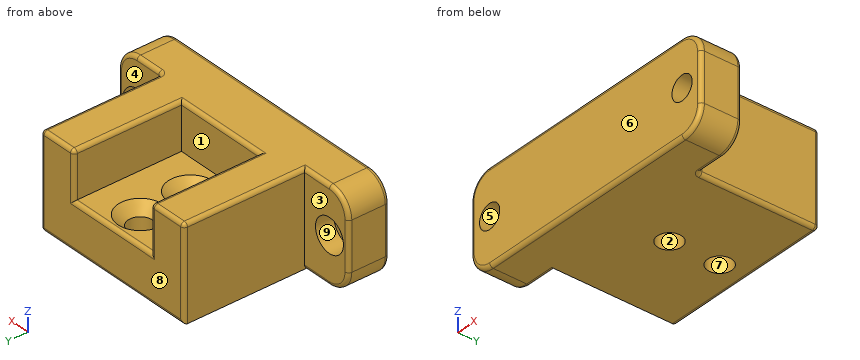
from build123d import *

# Parameters (mm, degrees)
BOSS_EXTRUDE1_DEPTH = 50
SKETCH2_W           = 50
SKETCH2_H           = 25
CUT_EXTRUDE2_DEPTH  = 58
SKETCH3_R           = 6.5
CUT_EXTRUDE3_DEPTH  = 58
SKETCH3_3_R         = 9
SKETCH3_3_R_2       = 6.5
CUT_EXTRUDE4_DEPTH  = 10
SKETCH6_R           = 6.5
CUT_EXTRUDE5_DEPTH  = 19.5
CUT_EXTRUDE9_START  = -19.5
SKETCH6_3_R         = 6.5
CUT_EXTRUDE9_DEPTH  = 8.5
CUT_EXTRUDE9_TAPER  = -45
FILLET1_R           = 12
FILLET2_R           = 2


with BuildPart() as part:
    # Sketch1 → Boss-Extrude1 (new body)
    with BuildSketch(Plane.XY):
        Polygon((74, 0), (-74, 0), (-74, 22), (-46, 22), (-46, 87), (46, 87), (46, 22), (74, 22), align=None)
    extrude(amount=BOSS_EXTRUDE1_DEPTH)

    # Sketch2 → Cut-Extrude2 (cut)
    with BuildSketch(Plane(origin=(0, 87, 0), x_dir=(1, 0, 0), z_dir=(0, 1, 0))):
        with Locations((0, -37.5)):
            Rectangle(SKETCH2_W, SKETCH2_H)
    extrude(amount=-CUT_EXTRUDE2_DEPTH, mode=Mode.SUBTRACT)

    # Sketch3 → Cut-Extrude3 (cut)
    with BuildSketch(Plane(origin=(0, 22, 0), x_dir=(1, 0, 0), z_dir=(0, 1, 0))):
        with Locations((62, -25)):
            Circle(SKETCH3_R)
    cut_extrude3 = extrude(amount=-CUT_EXTRUDE3_DEPTH, mode=Mode.SUBTRACT)

    # Sketch3_3 → Cut-Extrude4 (cut)
    with BuildSketch(Plane(origin=(0, 22, 0), x_dir=(1, 0, 0), z_dir=(0, 1, 0))):
        with Locations((62, -25)):
            Circle(SKETCH3_3_R)
        with Locations((62, -25)):
            Circle(SKETCH3_3_R_2, mode=Mode.SUBTRACT)
    cut_extrude4 = extrude(amount=-CUT_EXTRUDE4_DEPTH, mode=Mode.SUBTRACT)

    # Mirror2: Cut-Extrude3, Cut-Extrude4 across plane
    add(cut_extrude3.mirror(Plane(origin=(0, 0, 0), x_dir=(0, 0, 1), z_dir=(1, 0, 0))), mode=Mode.SUBTRACT)
    add(cut_extrude4.mirror(Plane(origin=(0, 0, 0), x_dir=(0, 0, 1), z_dir=(1, 0, 0))), mode=Mode.SUBTRACT)

    # Sketch6 → Cut-Extrude5 (cut)
    with BuildSketch(Plane(origin=(0, 0, 0), x_dir=(-1, 0, 0), z_dir=(0, 0, -1))):
        with Locations((0, 72)):
            Circle(SKETCH6_R)
    cut_extrude5 = extrude(amount=-CUT_EXTRUDE5_DEPTH, mode=Mode.SUBTRACT)

    # Sketch6_3 → Cut-Extrude9 (cut)
    with BuildSketch(Plane(origin=(0, 0, 0), x_dir=(-1, 0, 0), z_dir=(0, 0, -1)).offset(CUT_EXTRUDE9_START)):
        with Locations((0, 72)):
            Circle(SKETCH6_3_R)
    cut_extrude9 = extrude(amount=-CUT_EXTRUDE9_DEPTH, taper=CUT_EXTRUDE9_TAPER, mode=Mode.SUBTRACT)

    # Mirror3: Cut-Extrude5, Cut-Extrude9 across plane
    add(cut_extrude5.mirror(Plane.ZX.offset(58.5)), mode=Mode.SUBTRACT)
    add(cut_extrude9.mirror(Plane.ZX.offset(58.5)), mode=Mode.SUBTRACT)

    # Fillet1
    fillet1_edges = [part.edges().sort_by_distance(p)[0] for p in [
        (-74, 11, 0),
        (-74, 11, 50),
        (74, 11, 50),
        (74, 11, 0),
    ]]
    fillet(fillet1_edges, radius=FILLET1_R)

    # Fillet2
    fillet2_edges = [part.edges().sort_by_distance(p)[0] for p in [
        (-54, 22, 0),
        (-46, 87, 25),
        (46, 87, 25),
        (46, 22, 25),
        (-35.5, 87, 50),
        (25, 87, 37.5),
        (0, 29, 50),
        (25, 58, 50),
        (46, 54.5, 50),
        (-25, 58, 50),
        (0, 87, 25),
        (-25, 87, 37.5),
        (35.5, 87, 50),
        (-46, 54.5, 50),
        (-74, 0, 25),
        (-74, 22, 25),
        (0, 0, 0),
        (74, 0, 25),
        (0, 0, 50),
        (70.485281374, 0, 46.485281374),
        (70.485281374, 0, 3.514718626),
        (-70.485281374, 0, 46.485281374),
        (-70.485281374, 0, 3.514718626),
        (54, 22, 0),
        (0, 87, 0),
        (-70.485281374, 22, 46.485281374),
        (-70.485281374, 22, 3.514718626),
        (54, 22, 50),
        (74, 22, 25),
        (70.485281374, 22, 46.485281374),
        (-54, 22, 50),
        (46, 54.5, 0),
        (70.485281374, 22, 3.514718626),
    ]]
    fillet(fillet2_edges, radius=FILLET2_R)


solid = part.part
Can you work these out from the model? Positions are in its coordinate system, mm. Face numbers are marked on the shaded views. A direction names the side the tool comes from. Coordinates: 2 decimals unless noted, no trailing zeros. Order: outer loops, then holes, each group sorted by start corner. A loop starts at its lowest first (then second) coordinate and runs counter-clockwise, first axis right, second up. Notation, with made-up numbers: M 62.5,53 L 103.5,53 A35 cw 103.5,90 Z; hole C -28.75,58 d3. An arc over 180 degrees is marked long. Write item = value, one per line.
(1) Suppose I cut it at C-C on x = 23.5. Please give me the cut outline in (y, z), plus the area to 3 significant figures.
Results are:
outline = M 0,2 A2 ccw 2,0 L 85,0 A2 ccw 87,2 L 87,23 A2 ccw 85,25 L 29,25 L 29,48 A2 ccw 27,50 L 2,50 A2 ccw 0,48 Z
area = 2,900 mm2
(2) Suppose I cut it at B-B on y = 13.5. Please give me the cut outline in (x, z), plus the area to 3 significant figures.
Results are:
outline = M -74,12 A12 ccw -62,0 L 62,0 A12 ccw 74,12 L 74,38 A12 ccw 62,50 L -62,50 A12 ccw -74,38 Z; hole C -62,25 d18; hole C 62,25 d18
area = 6,770 mm2
(3) Suppose I cut it at A-A on x = 0. Please give me the cut outline in (y, z).
Results are:
outline = M 0,2 A2 ccw 2,0 L 38.5,0 L 38.5,19.5 L 33,25 L 29,25 L 29,48 A2 ccw 27,50 L 2,50 A2 ccw 0,48 Z; M 51.5,0 L 65.5,0 L 65.5,19.5 L 60,25 L 57,25 L 51.5,19.5 Z; M 78.5,0 L 85,0 A2 ccw 87,2 L 87,23 A2 ccw 85,25 L 84,25 L 78.5,19.5 Z
(4) If we mould it in two halves opening along Y, with no side actions, what happens to the marked faces 6, 7, 8 and 9? For each: pulls with the +Y half, pulls with the -Y half, needs draft (parallel to the pull), parting line crosses it, or undercut.
Results are:
face_6 = pulls with the -Y half
face_7 = undercut
face_8 = pulls with the +Y half
face_9 = needs draft
(5) I need wall thicknesses on line 1 along Y through (x, z) = (0, 15.5); line 2 along X through (y, z) = (5, 25); line 3 along X through (y, z) = (15.75, 25). Which ranges of each line are inside material? Lowest first, please. Write a range as [from, to].
Results are:
line_1 = [0, 38.5], [51.5, 65.5], [78.5, 87]
line_2 = [-74, -68.5], [-55.5, 55.5], [68.5, 74]
line_3 = [-74, -71], [-53, 53], [71, 74]
(6) For pin 1 Ø18.5 at (y, z) = (55.5, 37) entering from -X; pin 2 Ø9 at (x, z) = (66, 24) entering from +Y; pin 3 Ø23 at (y, z) = (64, 15.5) entering from +X; pin 4 Ø12 at (x, y) = (-3, 57) entering from -Z, each with a flat end and sliding along its axis, tell me the tip position at first contact or that it passes through.
Results are:
pin_1 = -46
pin_2 = 12
pin_3 = 46
pin_4 = 0
(7) For the marked faces 1, 2, 3, 4 and 5, which set-ups out of +Z, -Z, +X, -X, +Y, -Y let a thin tool reach every point of the face, with its end or its side?
Results are:
face_1 = +Z, +Y
face_2 = +Z, -Z
face_3 = +Z, -Z, -X, +Y
face_4 = +Z, -Z, +X, +Y
face_5 = +Y, -Y
